from build123d import *

# Parameters (mm, degrees)
BOSS_EXTRUDE1_DEPTH = 40


with BuildPart() as part:
    # Sketch1 → Boss-Extrude1 (new body)
    with BuildSketch(Plane(origin=(0, 0, 0), x_dir=(1, 0, 0), z_dir=(0, 1, 0))):
        with BuildLine():
            Line((1.45, 17.941502167), (1.45, 15))
            Line((1.45, 15), (-1.45, 15))
            Line((-1.45, 15), (-1.45, 17.941502167))
            ThreePointArc((-1.45, 17.941502167), (-12.204507364, -13.230646243), (18, 0))
            ThreePointArc((18, 0), (13.230646243, 12.204507364), (1.45, 17.941502167))
        make_face()
    extrude(amount=BOSS_EXTRUDE1_DEPTH)


solid = part.part
Verification items for the finished model (mm, model axes). A direction names the side the tool comes from. Coordinates: 2 decimals unless noted, no trailing zeros. Order: outer loops, then holes, each group sorted by start corner. A loop starts at its lowest first (then second) coordinate and runs counter-clockwise, first axis right, second up.
Item 1: Depth check by flat-ended pin: pin 1 (3 mm diameter, centred on y = 20.5, z = 13.5, fed in from +X); pin 2 (3 mm diameter, centred on y = 7.5, z = -13, fed in from -X); pin 3 (8 mm diameter, centred on x = -9, y = 26.5, fed in from +Z); pin 4 (5 mm diameter, centred on x = -3.5, z = 3.5, fed in from -Y). Enter the tip coordinate at first touch or a pass-through.
Filled in:
pin 1: stops at x = 13.42
pin 2: stops at x = -13.85
pin 3: stops at z = 17.29
pin 4: stops at y = 0
Item 2: Section check A-A, the plane z = -16. Enter the section's corners in (x, y), then the cut area to 3 significant figures.
Filled in:
outline: (-8.25, 0) - (-1.45, 0) - (-1.45, 40) - (-8.25, 40) - close; (1.45, 0) - (8.25, 0) - (8.25, 40) - (1.45, 40) - close
area: 544 mm2
Item 3: Section check D-D, the plane z = 10. Enter the section's corners in (x, y).
Filled in:
outline: (-14.97, 0) - (14.97, 0) - (14.97, 40) - (-14.97, 40) - close
Item 4: Section check C-C, the plane x = 0. Enter the section's corners in (y, z).
Filled in:
outline: (0, -15) - (40, -15) - (40, 18) - (0, 18) - close
Item 5: Access from +Z, -Z, +X, -X, +Y, -Y to the whole of each face (thin tool, end or side, straight path). Record for faces 1 (the face through (-1.45, 20, -16)), 2 (the face through (0, 0, 0)).
Filled in:
face 1: -Z, +Y, -Y
face 2: +Z, -Z, +X, -X, -Y
Item 6: Release check for a two-part mould opening along X. For faces 3 (the face through (0, 20, -15)), 4 (the face through (0, 40, 0)) record: +X half, -X half, draft (parallel to the pull), parting line (faces both ways), or undercut.
Filled in:
face 3: undercut
face 4: draft
Item 7: Material ranges on L1, parallel to X at y = 17.5, z = 0.5; L2, parallel to Z at x = -16, y = 9.5; L3, parallel to X at y = 22, z = -9, recorded low to high.
Filled in:
L1: x = -17.99 to 17.99
L2: z = -8.25 to 8.25
L3: x = -15.59 to 15.59
Item 8: Section check B-B, the plane y = 10. Enter the section's corners in (x, z), then the cut area to 3 significant figures.
Filled in:
outline: (-1.45, -17.94) - (-1.45, -15) - (1.45, -15) - (1.45, -17.94) arc R18 ccw (long way) to start
area: 1,010 mm2
